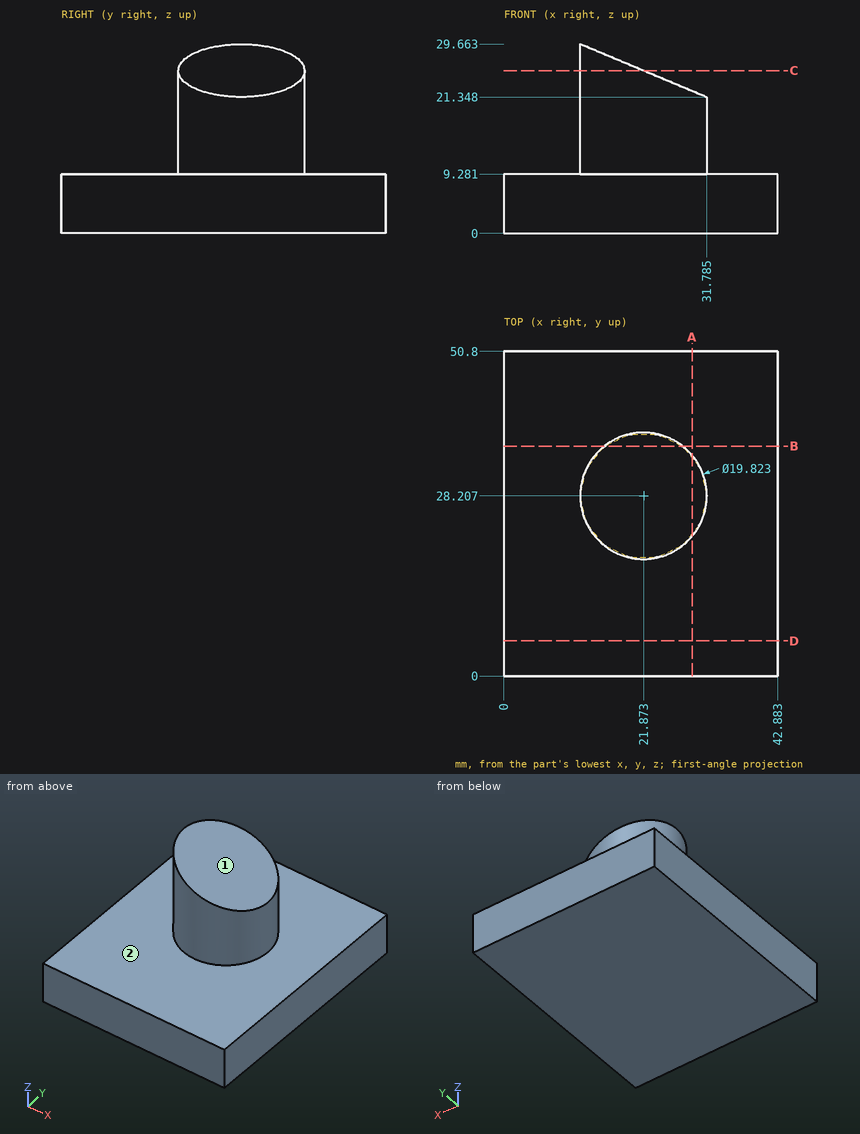
The drawing under review shows one solid part. Ordinate dimensions are in mm from its lowest x, y, z. A direction names the side the tool comes from. Round coordinates to 2 decimals unless told otherwise and drop trailing zeros. Write each loop counter-clockwise with the first axis right and the second up, starting at its lowest first coordinate (ties: lowest second). Pieces come first, ordered by that corner, then holes. Notation, with made-up numbers: (45, -31) - (95, -31) arc R15 ccw to (95, -3) - close; hole circle Ø9 at (24, 41). An arc over 180 degrees is marked (long way). Use one line per item in the form item = value.
Q1. Consider section B-B (y = 36). State the section outline as (x, z) points (1 decimal), and give its area (3 significant figures).
Answer key:
outline = (0, 0) - (42.9, 0) - (42.9, 9.3) - (28, 9.3) - (28, 22.9) - (15.7, 28.1) - (15.7, 9.3) - (0, 9.3) - close
area = 597 mm2
Q2. Insertion check: pin 1 Ø5 at (x, z) = (33.5, 12.5) entering from -Y (1 decimal); pin 2 Ø12 at (x, z) = (37.5, 11) entering from +Y; pin 3 Ø1.5 at (y, z) = (23.5, 14) entering from -X (1 decimal); pin 4 Ø10 at (y, z) = (36, 22.5) entering from -X. Each pin has a flat end and moves straight along its axis. Give the tip position at first contact, or say it passes through.
Answer key:
pin_1 = 24.3
pin_2 = 50.8
pin_3 = 12.8
pin_4 = 12.36
Q3. Consider section A-A (x = 29.5). State the section outline as (y, z) points, and give its area (3 significant figures).
Answer key:
outline = (0, 0) - (50.8, 0) - (50.8, 9.28) - (34.54, 9.28) - (34.54, 22.31) - (21.88, 22.31) - (21.88, 9.28) - (0, 9.28) - close
area = 636 mm2
Q4. Consider section C-C (z = 25.5). State the section outline as (x, y) points (1 decimal).
Answer key:
outline = (21.9, 18.3) - (21.9, 38.1) arc R9.9 ccw to start
Q5. Tool access review of the marked faces 1 and 2: name each direction out of +Z, -Z, +X, -X, +Y, -Y from which nothing blocks a thin tool from reaching the whole face with its end or side.
Answer key:
face_1 = +Z, +X, +Y, -Y
face_2 = +Z
Q6. For line 1 (Z direction, x = 30.5, y = 16); line 2 (Y direction, x = 18.5, z = 25.25); line 3 (X direction, y = 30, z = 24) (1 decimal), list the stretches that pass through material, from the lowest coordinate up. Write a range as [from, to].
Answer key:
line_1 = [0, 9.28]
line_2 = [18.89, 37.53]
line_3 = [12.1, 25.5]
Q7. Consider section D-D (y = 5.5). State the section outline as (x, z) points.
Answer key:
outline = (0, 0) - (42.88, 0) - (42.88, 9.28) - (0, 9.28) - close
